Source: CAD feature listing. Evaluate the final solid. Frame: model axes, mm. A direction names the side the tool comes from. Coordinates: 2 decimals unless noted, no trailing zeros. Write each loop counter-clockwise with the first axis right and the second up, starting at its lowest first coordinate (ties: lowest second). Pieces come first, ordered by that corner, then holes. Notation, with made-up numbers: (-28, -4.5) -> (-18, -4.5) arc R17 ccw to (-18, 13.5) -> close; hole circle Ø7 at (51, 6.25). An arc over 180 degrees is marked (long way). One line per item, written item: value. Start each with the question number.
1. First-contact query: P1, Ø1, axis at x = -18.5, z = 3, coming from the +Y side. Flat tip, straight axial feed; report the tip coordinate or a pass-through.
2. Access query for faces 4 (the flat face through (-8.89, -25, 2)), 5 (the cylindrical face through (-10.637, -86.861, 2.348)), 6 (the cylindrical face through (-15.19, -124.743, 2.348)). Directions: +Z, -Z, +X, -X, +Y, -Y. A direction counts if a zero-diameter tool reaches every point of the face in a straight line with its end or side. Return the directions, or none.
3. Section query A-A, the plane y = -17. Output: boundary loops of the cut face in (x, z).
4. Section query B-B, the plane z = 3.6. State how many separate pieces and enclosed holes the cut face has, and give its area (3 significant figures).
5. Mould query, pull axis Y, two halves, no side actions, for faces 1 (the flat face through (-19, -57, 0)), 2 (the cylindrical face through (-14.98, -47.32, 2.35)), 3 (the cylindrical face through (-18.743, 9.317, 2.348)). Classes: released by +Y, released by -Y, zero draft, split by the parting line, or undercut.
6. Section query D-D, the plane y = -62. Output: boundary loops of the cut face in (x, z), and give its area (3 significant figures).
7. Section query C-C, the plane x = -4. Output: boundary loops of the cut face in (y, z).
8. Line query: line 1 (X direction, y = -26.5, z = 2.15); line 2 (Y direction, x = -14, z = 3.2); line 3 (X direction, y = -64.5, z = 3.6). Output: solid intervals per line, ascending.
from build123d import *

# Parameters (mm, degrees)
SKETCH1_R           = 2.032
SKETCH1_W           = 20.32
SKETCH1_H           = 40.386
BOSS_EXTRUDE1_DEPTH = 4.7625
FILLET1_R           = 1.016
FILLET2_R           = 0.508


with BuildPart() as part:
    # Sketch1 → Boss-Extrude1 (new body)
    with BuildSketch(Plane.XY):
        with BuildLine():
            Line((0, -49.992035626), (0, 0))
            ThreePointArc((0, 0), (-19.05, 9.319382187), (-38.1, 0))
            Line((-38.1, 0), (-38.1, -24.996017813))
            ThreePointArc((-38.1, -24.996017813), (-32.885821078, -75.953581503), (-17.459395355, -124.799117107))
            ThreePointArc((-17.459395355, -124.799117107), (-15.078767061, -124.73890948), (-12.7, -124.627180771))
            ThreePointArc((-12.7, -124.627180771), (-10.590712033, -86.588003883), (0, -49.992035626))
        make_face()
        with Locations(Location((-14.0462, -0.866017813, 0), (0, 0, 180))):
            Circle(SKETCH1_R, mode=Mode.SUBTRACT)
        with Locations(Location((-24.0538, -0.866017813, 0), (0, 0, 180))):
            Circle(SKETCH1_R, mode=Mode.SUBTRACT)
        with Locations(Location((-24.0538, -49.126017813, 0), (0, 0, 180))):
            Circle(SKETCH1_R, mode=Mode.SUBTRACT)
        with Locations(Location((-14.0462, -49.126017813, 0), (0, 0, 180))):
            Circle(SKETCH1_R, mode=Mode.SUBTRACT)
        with Locations((-19.05, -24.996017813)):
            Rectangle(SKETCH1_W, SKETCH1_H, mode=Mode.SUBTRACT)
    extrude(amount=BOSS_EXTRUDE1_DEPTH)

    # Fillet1
    fillet1_edges = [part.edges().sort_by_distance(p)[0] for p in [
        (-8.89, -45.189017813, 2.38125),
        (-8.89, -4.803017813, 2.38125),
        (-29.21, -4.803017813, 2.38125),
        (-29.21, -45.189017813, 2.38125),
    ]]
    fillet(fillet1_edges, radius=FILLET1_R)

    # Fillet2
    fillet2_edges = [part.edges().sort_by_distance(p)[0] for p in [
        (-12.7, -124.627180771, 2.38125),
        (-17.459395355, -124.799117107, 2.38125),
    ]]
    fillet(fillet2_edges, radius=FILLET2_R)


solid = part.part
Computed values:
1. P1: stops at y = 9.32
2. face 4: +Z, -Z
2. face 5: +Z, -Z, +X
2. face 6: +Z, -Z, +X, -Y
3. outline: (-38.1, 0) -> (-29.21, 0) -> (-29.21, 4.76) -> (-38.1, 4.76) -> close; (-8.89, 0) -> (0, 0) -> (0, 4.76) -> (-8.89, 4.76) -> close
4. separate pieces: 1
4. enclosed holes: 5
4. area: 2,760 mm²
5. face 1: zero draft
5. face 2: undercut
5. face 3: released by +Y
6. outline: (-35.36, 0) -> (-4.48, 0) -> (-4.48, 4.76) -> (-35.36, 4.76) -> close
6. area: 147 mm²
7. outline: (-60.58, 0) -> (4.05, 0) -> (4.05, 4.76) -> (-60.58, 4.76) -> close
8. line 1: x = -38.1 to -29.21, -8.89 to 0
8. line 2: y = -124.69 to -51.16, -47.09 to -45.19, -4.8 to -2.9, 1.17 to 8.79
8. line 3: x = -34.98 to -5.28
